```python
from build123d import *

# Parameters (mm, degrees)
F1_DEPTH  = 2
F3_DEPTH  = 3
F5_DEPTH  = 2
F7_DEPTH  = 3
F8_R      = 0.99999
F9_W      = 24
F9_H      = 22.6653645039
F10_DEPTH = 10
F11_W     = 24
F11_H     = 25
F11_W_2   = 8
F11_H_2   = 8
F12_DEPTH = 3
F13_R     = 1
F14_W     = 24
F14_H     = 13.6653645039
F15_DEPTH = 2


# Not quite as in the source:
# - a fillet or chamfer is up to 0.001 mm smaller than in the source, because OpenCascade refuses the exact size


with BuildPart() as f1:
    # F0 (on Top) → F1 (new body)
    with BuildSketch(Plane.XY):
        with BuildLine():
            ThreePointArc((5.5, 1.5), (0, 24.1653645039), (-5.5, 1.5))
            Line((-5.5, 1.5), (-5.5, -1.5))
            ThreePointArc((-5.5, -1.5), (0, -24.1653645039), (5.5, -1.5))
            Line((5.5, -1.5), (5.5, 1.5))
        make_face()
    extrude(amount=F1_DEPTH)

    # F2 (on face) → F3 (join)
    with BuildSketch(Plane.XY.offset(2)):
        with BuildLine():
            Line((9.7844830762, 19.1125863177), (8.6602540378, 17.1653645039))
            ThreePointArc((8.6602540378, 17.1653645039), (9.4991255677, 9.0402063559), (4, 3.0002131139))
            Line((4, 3.0002131139), (4, -6.2432010007))
            Line((4, -6.2432010007), (9.1651513899, -16.1653645039))
            ThreePointArc((9.1651513899, -16.1653645039), (9.5868378212, -9.3206253964), (5.5, -3.8137179596))
            Line((5.5, -3.8137179596), (5.5, 1.5))
            ThreePointArc((5.5, 1.5), (11.6599594736, 9.3289327537), (9.7844830762, 19.1125863177))
        make_face()
        with BuildLine():
            ThreePointArc((-4, 3.0002131139), (-9.4991255677, 9.0402063559), (-8.6602540378, 17.1653645039))
            Line((-8.6602540378, 17.1653645039), (-9.7844830762, 19.1125863177))
            ThreePointArc((-9.7844830762, 19.1125863177), (-11.6599594736, 9.3289327537), (-5.5, 1.5))
            Line((-5.5, 1.5), (-5.5, -3.8137179596))
            ThreePointArc((-5.5, -3.8137179596), (-9.5868378212, -9.3206253964), (-9.1651513899, -16.1653645039))
            Line((-9.1651513899, -16.1653645039), (-4, -6.2432010007))
            Line((-4, -6.2432010007), (-4, 3.0002131139))
        make_face()
    extrude(amount=F3_DEPTH)

    # F4 (on face) → F5 (join)
    with BuildSketch(Plane.XY.offset(5)):
        with BuildLine():
            Line((-8.0717844057, 16.1461052023), (-9.7844830762, 19.1125863177))
            ThreePointArc((-9.7844830762, 19.1125863177), (-11.6599594736, 9.3289327537), (-5.5, 1.5))
            Line((-5.5, 1.5), (-5.5, -5.0414610795))
            ThreePointArc((-5.5, -5.0414610795), (-8.6043935433, -9.5263473097), (-8.5483759414, -14.980549891))
            Line((-8.5483759414, -14.980549891), (-4, -6.2432010007))
            Line((-4, -6.2432010007), (-4, 4.1031067556))
            ThreePointArc((-4, 4.1031067556), (-8.5258693153, 9.2827350759), (-8.0717844057, 16.1461052023))
        make_face()
        with BuildLine():
            ThreePointArc((5.5, 1.5), (11.6599594736, 9.3289327537), (9.7844830762, 19.1125863177))
            Line((9.7844830762, 19.1125863177), (8.0717844057, 16.1461052023))
            ThreePointArc((8.0717844057, 16.1461052023), (8.5258693153, 9.2827350759), (4, 4.1031067556))
            Line((4, 4.1031067556), (4, -6.2432010007))
            Line((4, -6.2432010007), (8.5483759414, -14.980549891))
            ThreePointArc((8.5483759414, -14.980549891), (8.6043935433, -9.5263473097), (5.5, -5.0414610795))
            Line((5.5, -5.0414610795), (5.5, 1.5))
        make_face()
    extrude(amount=F5_DEPTH)

    # F6 (on face) → F7 (join)
    with BuildSketch(Plane.XY.offset(7)):
        with BuildLine():
            Line((9.7844830762, 19.1125863177), (8.6602540378, 17.1653645039))
            ThreePointArc((8.6602540378, 17.1653645039), (9.4991255677, 9.0402063559), (4, 3.0002131139))
            Line((4, 3.0002131139), (4, -6.2432010007))
            Line((4, -6.2432010007), (9.1651513899, -16.1653645039))
            ThreePointArc((9.1651513899, -16.1653645039), (9.5868378212, -9.3206253964), (5.5, -3.8137179596))
            Line((5.5, -3.8137179596), (5.5, 1.5))
            ThreePointArc((5.5, 1.5), (11.6599594736, 9.3289327537), (9.7844830762, 19.1125863177))
        make_face()
        with BuildLine():
            ThreePointArc((-4, 3.0002131139), (-9.4991255677, 9.0402063559), (-8.6602540378, 17.1653645039))
            Line((-8.6602540378, 17.1653645039), (-9.7844830762, 19.1125863177))
            ThreePointArc((-9.7844830762, 19.1125863177), (-11.6599594736, 9.3289327537), (-5.5, 1.5))
            Line((-5.5, 1.5), (-5.5, -3.8137179596))
            ThreePointArc((-5.5, -3.8137179596), (-9.5868378212, -9.3206253964), (-9.1651513899, -16.1653645039))
            Line((-9.1651513899, -16.1653645039), (-4, -6.2432010007))
            Line((-4, -6.2432010007), (-4, 3.0002131139))
        make_face()
    extrude(amount=F7_DEPTH)

    # F8 (radius 1 in the source; OpenCascade refuses exactly that, so slightly less here)
    f8_edges = [f1.edges().sort_by_distance(p)[0] for p in [
        (8.525869, 9.282735, 7),
        (-8.525869, 9.282735, 7),
        (-8.525869, 9.282735, 5),
        (8.525869, 9.282735, 5),
        (-8.604394, -9.526347, 5),
        (-8.604394, -9.526347, 7),
        (8.604394, -9.526347, 7),
        (8.604394, -9.526347, 5),
    ]]
    fillet(f8_edges, radius=F8_R)

    # F9 (on face) → F10 (cut)
    with BuildSketch(Plane.XY.offset(10)):
        with Locations((0, -12.8326822519)):
            Rectangle(F9_W, F9_H)
    extrude(amount=-F10_DEPTH, mode=Mode.SUBTRACT)

    # F11 (on face) → F12 (join)
    with BuildSketch(Plane.XZ.offset(1.5)):
        with Locations((0, 12.5)):
            Rectangle(F11_W, F11_H)
        with Locations((0, 6)):
            Rectangle(F11_W_2, F11_H_2, mode=Mode.SUBTRACT)
    extrude(amount=F12_DEPTH)

    # F13
    f13_edges = [f1.edges().sort_by_distance(p)[0] for p in [
        (0, -4.5, 10),
        (4, -4.5, 6),
        (0, -4.5, 2),
        (-4, -4.5, 6),
    ]]
    fillet(f13_edges, radius=F13_R)

    # F14 (on face) → F15 (join)
    with BuildSketch(Plane(origin=(0, 0, 0), x_dir=(1, 0, 0), z_dir=(0, 0, -1))):
        with Locations((0, -5.3326822519)):
            Rectangle(F14_W, F14_H)
    extrude(amount=-F15_DEPTH)


solid = f1.part
```
Geometry check sheet. Reference: the model listing, model coordinates, mm. A direction names the side the tool comes from. Round coordinates to 2 decimals unless told otherwise and drop trailing zeros. Order: outer loops, then holes, each group sorted by start corner. A loop starts at its lowest first (then second) coordinate and runs counter-clockwise, first axis right, second up. Notation, with made-up numbers: (-19.5, 83.25) - (23.5, 83.25) arc R18 cw to (23.5, 98.25) - close; hole circle Ø2 at (-25, 85.5). An arc over 180 degrees is marked (long way). Use a Markdown table: item, result. Add a question column.
(1) Release check for a two-part mould opening along X. For faces 4 (the flat face through (12, -2, 10)), 5 (the cylindrical face through (9.535, 9.152, 8.479)), 6 (the flat face through (-10, 2, 2)), 7 (the cylindrical face through (-4.301, -4.215, 6.07)) record: pulls with the +X half, pulls with the -X half, needs draft (parallel to the pull), parting line crosses it, or undercut.
(2) Sectioned sample at A-A, the plane x = 0. Enter the section's corners in (y, z), and give its area (3 significant figures).
(3) Tool access check on faces 1 (the cylindrical face through (0.07, -4.215, 10.301)), 2 (the flat face through (9.5, 8.1, 10)), 3 (the cylindrical face through (-9.462, 8.929, 8.479)). Record the directions out of +Z, -Z, +X, -X, +Y, -Y that give a thin tool (end or side, any length) a straight path to the whole face; none if there is none.
(4) Depth check by flat-ended pin: pin 1 (2.5 mm diameter, centred on y = 0.5, z = 6.5, fed in from -X); pin 2 (1.5 mm diameter, centred on y = 17.5, z = 12.5, fed in from -X); pin 3 (5 mm diameter, centred on x = 3.5, y = 17.5, fed in from +Z); pin 4 (3 mm diameter, centred on x = 9, y = 10, fed in from +Z). Enter the tip coordinate at first touch or a pass-through.
(5) Sectioned sample at B-B, the plane y = -2.25. Enter the section's corners in (x, z).
(6) Sectioned sample at C-C, the plane z = 22.25. Enter the section's corners in (x, y), and give its area (3 significant figures).
(7) Sectioned sample at D-D, the plane y = 21.5. Enter the section's corners in (x, z), and give its area (3 significant figures).
(8) Material ranges on line 1 along X through (y, z) = (-1.75, 3.5); line 2 along Z through (x, y) = (8, 12.5); line 3 along Y through (x, z) = (4.25, 17), recorded low to high. Write a range as [from, to].
Answers below:
| question | item | result |
|---|---|---|
| 1 | face 4 | pulls with the +X half |
| 1 | face 5 | undercut |
| 1 | face 6 | needs draft |
| 1 | face 7 | undercut |
| 2 | outline | (-4.5, 0) - (24.17, 0) - (24.17, 2) - (-3.5, 2) arc R1 ccw to (-4.5, 1) - close; (-4.5, 11) arc R1 ccw to (-3.5, 10) - (-1.5, 10) - (-1.5, 25) - (-4.5, 25) - close |
| 2 | area | 102 mm² |
| 3 | face 1 | -Y |
| 3 | face 2 | +Z, +X, -X, +Y |
| 3 | face 3 | +Z |
| 4 | pin 1 | x = -5.96 |
| 4 | pin 2 | through |
| 4 | pin 3 | z = 2 |
| 4 | pin 4 | z = 10 |
| 5 | outline | (-12, 0) - (12, 0) - (12, 25) - (-12, 25) - close; hole (-4, 2) - (4, 2) - (4, 10) - (-4, 10) - close |
| 6 | outline | (-12, -4.5) - (12, -4.5) - (12, -1.5) - (-12, -1.5) - close |
| 6 | area | 72.0 mm² |
| 7 | outline | (-7.54, 0) - (7.54, 0) - (7.54, 2) - (-7.54, 2) - close |
| 7 | area | 30.2 mm² |
| 8 | line 1 | [-12, -4], [4, 12] |
| 8 | line 2 | [0, 2] |
| 8 | line 3 | [-4.5, -1.5] |
